```python
from build123d import *

# Parameters (mm, degrees)
F2_DEPTH       = 3
F3_R           = 3
F4_DEPTH       = 1.2
F5_DEPTH       = 12.5
F6_W           = 2
F6_H           = 10
F7_DEPTH       = 5
F9_DEPTH       = 3
F10_SIZE       = 5
F11_T1_DEPTH   = 15.1433659759
F11_T3_DEPTH   = 15.1433659759
F11_T5_DEPTH   = 8
F11_T10_DEPTH  = 7.571682988
F11_T15_DEPTH  = 7.571682988
F11_T17_DEPTH  = 7.8722554791
F11_T19_DEPTH  = 31.6397752967
F11_T21_DEPTH  = 8.1433659759
F11_T23_DEPTH  = 28.997160307
F12_R          = 1.5
F13_DEPTH      = 37.001
F13_DEPTH_BACK = 12.001


# Not quite as in the source:
# - a fillet or chamfer that OpenCascade refuses, or shapes differently, is made with other operations: its cross-section is extruded or revolved along the edge and cut away or added


with BuildPart() as f2:
    # F0 (on Top) → F2 (new body)
    with BuildSketch(Plane.XY):
        with BuildLine():
            ThreePointArc((20.5, -4), (16.5, 0), (20.5, 4))
            Line((20.5, 4), (-20.5, 4))
            ThreePointArc((-20.5, 4), (-17.6715728753, 2.8284271247), (-16.5, 0))
            ThreePointArc((-16.5, 0), (-17.6715728753, -2.8284271247), (-20.5, -4))
            Line((-20.5, -4), (20.5, -4))
        make_face()
        with BuildLine():
            ThreePointArc((24.5, 0), (23.3284271247, 2.8284271247), (20.5, 4))
            Line((20.5, 4), (20.5, 1.75))
            ThreePointArc((20.5, 1.75), (21.7374368671, 1.2374368671), (22.25, 0))
            ThreePointArc((22.25, 0), (21.7374368671, -1.2374368671), (20.5, -1.75))
            Line((20.5, -1.75), (20.5, -4))
            ThreePointArc((20.5, -4), (23.3284271247, -2.8284271247), (24.5, 0))
        make_face()
        with BuildLine():
            Line((20.5, 1.75), (20.5, 4))
            ThreePointArc((20.5, 4), (16.5, 0), (20.5, -4))
            Line((20.5, -4), (20.5, -1.75))
            ThreePointArc((20.5, -1.75), (18.75, 0), (20.5, 1.75))
        make_face()
        with BuildLine():
            ThreePointArc((-16.5, 0), (-17.6715728753, 2.8284271247), (-20.5, 4))
            Line((-20.5, 4), (-20.5, 1.75))
            ThreePointArc((-20.5, 1.75), (-19.2625631329, 1.2374368671), (-18.75, 0))
            ThreePointArc((-18.75, 0), (-19.2625631329, -1.2374368671), (-20.5, -1.75))
            Line((-20.5, -1.75), (-20.5, -4))
            ThreePointArc((-20.5, -4), (-17.6715728753, -2.8284271247), (-16.5, 0))
        make_face()
        with BuildLine():
            Line((-20.5, 1.75), (-20.5, 4))
            ThreePointArc((-20.5, 4), (-24.5, 0), (-20.5, -4))
            Line((-20.5, -4), (-20.5, -1.75))
            ThreePointArc((-20.5, -1.75), (-22.25, 0), (-20.5, 1.75))
        make_face()
    extrude(amount=F2_DEPTH)

    # F3 (on face) → F4 (cut)
    with BuildSketch(Plane.XY.offset(3)):
        with Locations((-20.5, 0)):
            Circle(F3_R)
        with Locations((20.5, 0)):
            Circle(F3_R)
    extrude(amount=-F4_DEPTH, mode=Mode.SUBTRACT)

    # F1 (on Right) → F5 (join, symmetric)
    with BuildSketch(Plane.YZ):
        Polygon((-14.454310627, 0), (0, 0), (4, 0), (4, 7.0531719961), (1.1022225211, 7.8296291314), (-0.1918727044, 3), (-9.8511309673, 5.588190451), (-7.2629405162, 15.2474487139), (-10.1607179951, 16.0239058492), align=None)
    extrude(amount=F5_DEPTH, both=True)

    # F6 (on face) → F7 (join, through all)
    with BuildSketch(Plane(origin=(0, 0.737146966, 2.7510699296), x_dir=(1, 0, 0), z_dir=(0, 0.2588190451, 0.9659258263))):
        with Locations((11.5, -5.9617919358)):
            Rectangle(F6_W, F6_H)
        with Locations((-11.5, -5.9617919358)):
            Rectangle(F6_W, F6_H)
    extrude(amount=F7_DEPTH)

    # F8 (on face) → F9 (cut, through all)
    with BuildSketch(Plane(origin=(0, -13.4860554121, 3.6135776568), x_dir=(1, 0, 0), z_dir=(0, -0.9659258263, 0.2588190451))):
        with BuildLine():
            ThreePointArc((-8, 12.8481171687), (0, 4.8481171687), (8, 12.8481171687))
            Line((8, 12.8481171687), (-8, 12.8481171687))
        make_face()
    extrude(amount=-F9_DEPTH, mode=Mode.SUBTRACT)

    # F10
    f10_edges = [f2.edges().sort_by_distance(p)[0] for p in [
        (-12.5, -4, 1.5),
        (12.5, -4, 1.5),
    ]]
    chamfer(f10_edges, length=F10_SIZE)

    # F11: chamfer of 1 on 12 edges, made by hand

    # F11_s2 → F11_t1 (join)
    with BuildSketch(Plane(origin=(0, -13.0723329483, 3.5027210567), x_dir=(1, 0, 0), z_dir=(0, 0.9659258263, -0.2588190451))):
        Polygon((-9.5, -2.8481171687), (-10.5, -3.8481171687), (-10.5, -2.8481171687), align=None)
    extrude(amount=F11_T1_DEPTH)

    # F11_s4 → F11_t3 (join)
    with BuildSketch(Plane(origin=(0, 1.5550353448, -0.4166704648), x_dir=(1, 0, 0), z_dir=(0, -0.9659258263, 0.2588190451))):
        Polygon((9.5, 2.8481171687), (10.5, 3.8481171687), (10.5, 2.8481171687), align=None)
    extrude(amount=F11_T3_DEPTH)

    # F11_s6 → F11_t5 (join)
    with BuildSketch(Plane.XZ.offset(-4)):
        Polygon((12.5, 4), (13.5, 3), (12.5, 3), align=None)
        Polygon((-13.5, 3), (-12.5, 4), (-12.5, 3), align=None)
    extrude(amount=F11_T5_DEPTH)


with BuildPart() as f11_tool8:
    # F11_s9 → F11_t10 (new body)
    with BuildSketch(Plane.XZ.offset(4)):
        Polygon((-13.5, 3), (-12.5, 4), (-12.5, 3), align=None)
    extrude(amount=F11_T10_DEPTH)

    split(bisect_by=Plane(origin=(-10.75, -10.75, 0), x_dir=(0, 0, 1), z_dir=(0.7071067812, 0.7071067812, 0)), keep=Keep.TOP)


with BuildPart() as f2_1:
    add(f2.part)

    # F11_t7: union F11_tool8
    add(f11_tool8.part)


with BuildPart() as f11_tool13:
    # F11_s14 → F11_t15 (new body)
    with BuildSketch(Plane.XZ.offset(4)):
        Polygon((12.5, 4), (13.5, 3), (12.5, 3), align=None)
    extrude(amount=F11_T15_DEPTH)

    split(bisect_by=Plane(origin=(10.75, -10.75, 0), x_dir=(0, 0, 1), z_dir=(-0.7071067812, 0.7071067812, 0)), keep=Keep.TOP)


with BuildPart() as f2_2:
    add(f2_1.part)

    # F11_t12: union F11_tool13
    add(f11_tool13.part)

    # F11_s18 → F11_t17 (cut)
    with BuildSketch(Plane(origin=(0, -15.8391741119, 4.244093912), x_dir=(1, 0, 0), z_dir=(0, 0.9659258263, -0.2588190451))):
        with BuildLine():
            Line((-7.95046392, -11.9592282798), (-8.94427191, -12.8481171687))
            Line((-8.94427191, -12.8481171687), (-8, -12.8481171687))
            ThreePointArc((-8, -12.8481171687), (-7.9868043053, -12.3888166251), (-7.95046392, -11.9592282798))
        make_face()
        with BuildLine():
            Line((8.94427191, -12.8481171687), (7.95046392, -11.9592282798))
            ThreePointArc((7.95046392, -11.9592282798), (7.9868043053, -12.3888166251), (8, -12.8481171687))
            Line((8, -12.8481171687), (8.94427191, -12.8481171687))
        make_face()
    extrude(amount=F11_T17_DEPTH, mode=Mode.SUBTRACT)

    # F11_s20 → F11_t19 (cut)
    with BuildSketch(Plane.YZ.offset(-15.8198876484)):
        Polygon((-14.1170110805, 1.2588190451), (-13.1510852542, 0), (-14.454310627, 0), align=None)
    extrude(amount=F11_T19_DEPTH, mode=Mode.SUBTRACT)

    # F11_s22 → F11_t21 (cut)
    with BuildSketch(Plane(origin=(0, -8.1042229181, 2.1715199862), x_dir=(1, 0, 0), z_dir=(0, -0.9659258263, 0.2588190451))):
        Polygon((-12.5, 11.8481171687), (-11.5, 12.8481171687), (-12.5, 12.8481171687), align=None)
        Polygon((11.5, 12.8481171687), (12.5, 11.8481171687), (12.5, 12.8481171687), align=None)
    extrude(amount=F11_T21_DEPTH, mode=Mode.SUBTRACT)

    # F11_s24 → F11_t23 (cut)
    with BuildSketch(Plane.YZ.offset(-14.4985801535)):
        Polygon((4, 6.2858450082), (3.2588190451, 7.2517708344), (4, 7.0531719961), align=None)
    extrude(amount=F11_T23_DEPTH, mode=Mode.SUBTRACT)

    # F12 (on face) → F13 (cut, two sides)
    with BuildSketch(Plane(origin=(-12.5, 0, 0), x_dir=(0, -1, 0), z_dir=(-1, 0, 0))) as f13_sk:
        with Locations((10, 2)):
            Circle(F12_R)
    extrude(amount=-F13_DEPTH, mode=Mode.SUBTRACT)
    extrude(f13_sk.sketch, amount=F13_DEPTH_BACK, mode=Mode.SUBTRACT)


solid = f2_2.part
```
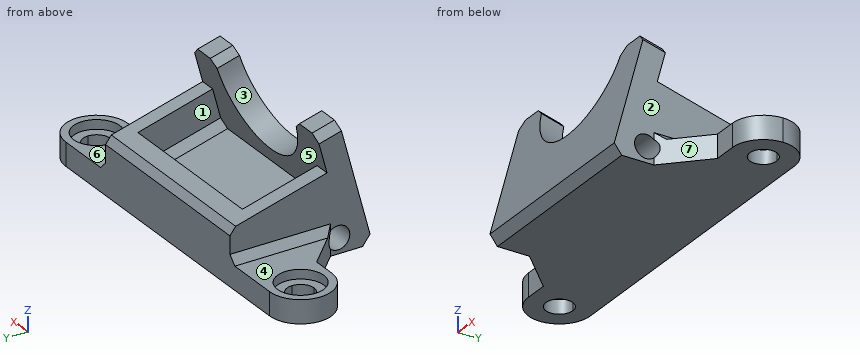
Check sheet for the modelled part. Datum: model origin and axes. Units: mm. Face numbers are marked on the shaded views. A direction names the side the tool comes from. Coordinates: 2 decimals unless noted, no trailing zeros. Write each loop counter-clockwise with the first axis right and the second up, starting at its lowest first coordinate (ties: lowest second). Pieces come first, ordered by that corner, then holes. Notation, with made-up numbers: (45.5, -37) -> (83.5, -37) arc R28 cw to (83.5, 0) -> close; hole circle Ø7 at (-20.5, 73.25). An arc over 180 degrees is marked (long way). Use a Markdown table: item, result.
1. Sectioned sample at C-C (x = 14). Enter the section's corners in (y, z), plus the area to 3 significant figures.
Reported:
| item | result |
|---|---|
| outline | (-7.5, 0) -> (4, 0) -> (4, 3) -> (-7.5, 3) -> close |
| area | 34.5 mm2 |
2. Sectioned sample at B-B (y = -6.5). Enter the section's corners in (x, z).
Reported:
| item | result |
|---|---|
| outline | (-15, 0) -> (15, 0) -> (15, 3) -> (13.5, 3) -> (12.5, 4) -> (12.5, 9.87) -> (10.5, 9.87) -> (10.5, 5.73) -> (9.5, 4.69) -> (-9.5, 4.69) -> (-10.5, 5.73) -> (-10.5, 9.87) -> (-12.5, 9.87) -> (-12.5, 4) -> (-13.5, 3) -> (-15, 3) -> close |
3. Tool access check on the marked faces 4, 5, 6 and 7. Record the directions out of +Z, -Z, +X, -X, +Y, -Y that give a thin tool (end or side, any length) a straight path to the whole face; none if there is none.
Reported:
| item | result |
|---|---|
| face 4 | +Z, -X, +Y, -Y |
| face 5 | none |
| face 6 | +Z, +X, +Y, -Y |
| face 7 | +Z, -Z, +X, -Y |
4. Scan lines: line 1 along X through (y, z) = (-6.5, 8); line 2 along Y through (x, z) = (-20.5, 2.8); line 3 along Z through (x, y) = (22, -3). Record each from-to range of solid material in increasing order.
Reported:
| item | result |
|---|---|
| line 1 | x = -12.5 to -10.5, 10.5 to 12.5 |
| line 2 | y = -4 to -3, 3 to 4 |
| line 3 | z = 0 to 3 |
5. Go/stop test with flat-tipped pins: pin 1 Ø2 at (x, y) = (17.5, -8) entering from -Z; pin 2 Ø3.5 at (x, z) = (-19.5, 2) entering from -Y; pin 3 Ø2.5 at (x, z) = (18.5, 2) entering from -Y; pin 4 Ø3 at (y, z) = (-2, 7) entering from +X. Record where each tip stops, or that it passes through.
Reported:
| item | result |
|---|---|
| pin 1 | passes through |
| pin 2 | stops at y = -4 |
| pin 3 | stops at y = -4.25 |
| pin 4 | stops at x = 12.5 |
6. Release check for a two-part mould opening along Z. For the marked faces 1, 2 and 3 record: pulls with the +Z half, pulls with the -Z half, needs draft (parallel to the pull), parting line crosses it, or undercut.
Reported:
| item | result |
|---|---|
| face 1 | undercut |
| face 2 | needs draft |
| face 3 | pulls with the +Z half |
7. Sectioned sample at A-A (y = -1). Give the number of separate pieces and of enclosed holes in the cut face, plus the area to 3 significant figures.
Reported:
| item | result |
|---|---|
| separate pieces | 3 |
| enclosed holes | 0 |
| area | 150 mm2 |
